Job drawing, mm, ordinate dimensions from the low corner. One solid piece. Round coordinates to 2 decimals unless told otherwise and drop trailing zeros. Loops run counter-clockwise (first coordinate to the right, second up) from the corner with the lowest first, then second, coordinate; pieces in that order, holes last.
1) Probe line 1 (Y direction, x = 470, z = 7); line 2 (X direction, y = 283, z = 4.75); line 3 (X direction, y = 620, z = 14). List the from-to ranges inside material, lowest first.
2) Band-saw the part on C-C, the plane z = 7. Write the cut outline in (x, y).
3) Band-saw the part on D-D, the plane x = 470. Write the cut outline in (y, z), then the cut area to 3 significant figures.
4) Band-saw the part on B-B, the plane x = 653. Write the cut outline in (y, z), then the cut area to 3 significant figures.
5) Band-saw the part on A-A, the plane y = 266. Write the cut outline in (x, z), then the cut area to 3 significant figures.
6) Drop a flat-ended pin along its axis: P1, Ø14, axis at x = 470, y = 620, coming from the -Z side. Give the stop position or say it passes through.
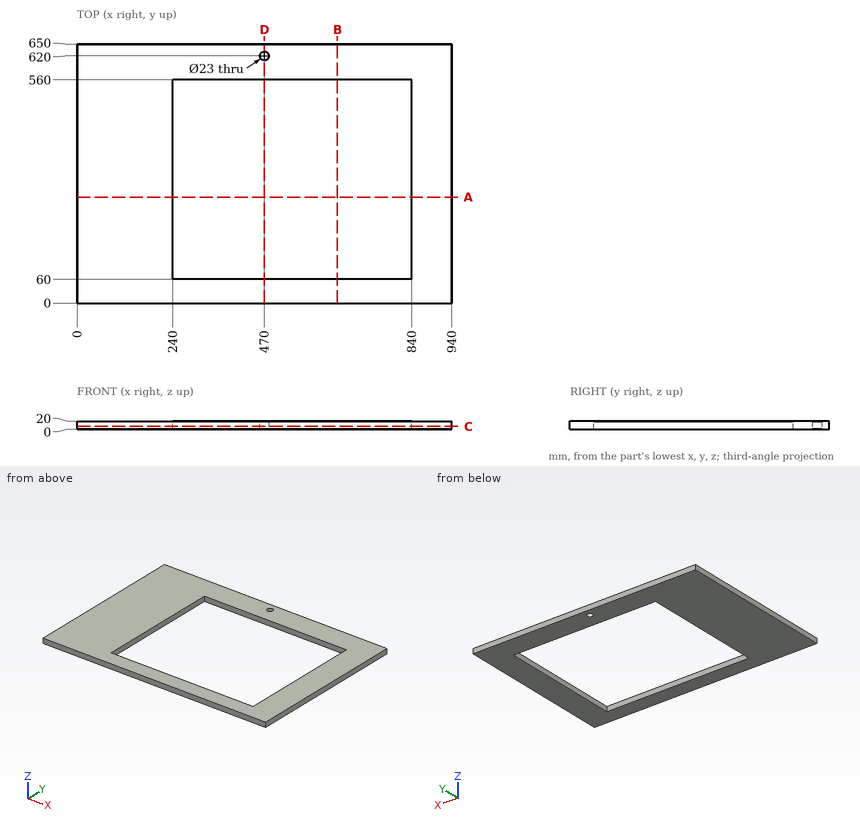
Reported:
1. line 1: y = 0 to 60, 560 to 608.5, 631.5 to 650
1. line 2: x = 0 to 240, 840 to 940
1. line 3: x = 0 to 458.5, 481.5 to 940
2. outline: (0, 0) - (940, 0) - (940, 650) - (0, 650) - close; hole (240, 60) - (840, 60) - (840, 560) - (240, 560) - close; hole circle Ø23 at (470, 620)
3. outline: (0, 0) - (60, 0) - (60, 20) - (0, 20) - close; (560, 0) - (608.5, 0) - (608.5, 20) - (560, 20) - close; (631.5, 0) - (650, 0) - (650, 20) - (631.5, 20) - close
3. area: 2,540 mm2
4. outline: (0, 0) - (60, 0) - (60, 20) - (0, 20) - close; (560, 0) - (650, 0) - (650, 20) - (560, 20) - close
4. area: 3,000 mm2
5. outline: (0, 0) - (240, 0) - (240, 20) - (0, 20) - close; (840, 0) - (940, 0) - (940, 20) - (840, 20) - close
5. area: 6,800 mm2
6. P1: passes through
